```python
from build123d import *

# Parameters (mm, degrees)
F0_W     = 88.9
F0_H     = 25.4
F1_DEPTH = 3.175
F2_R     = 3.5
F3_DEPTH = 10.16
F4_R     = 1.9685
F5_DEPTH = 25.4
F6_W     = 4.374
F6_H     = 25.4
F7_DEPTH = 20.32


with BuildPart() as f1:
    # F0 (on Top) → F1 (new body)
    with BuildSketch(Plane.XY):
        Rectangle(F0_W, F0_H)
    extrude(amount=F1_DEPTH)

    # F2 (on face) → F3 (join)
    with BuildSketch(Plane.XY.offset(3.175)):
        with Locations((40.95, 0)):
            Circle(F2_R)
    extrude(amount=F3_DEPTH)

    # F4 (on face) → F5 (cut)
    with BuildSketch(Plane.XY.offset(3.175)):
        with Locations((3.612, 0)):
            Circle(F4_R)
    extrude(amount=-F5_DEPTH, mode=Mode.SUBTRACT)

    # F6 (on face) → F7 (join)
    with BuildSketch(Plane.XY.offset(3.175)):
        with Locations((-42.263, 0)):
            Rectangle(F6_W, F6_H)
    extrude(amount=F7_DEPTH)


solid = f1.part
```
Build history of the part. All positions in model axes, mm. A direction names the side the tool comes from. Round coordinates to 2 decimals unless told otherwise and drop trailing zeros. Order: outer loops, then holes, each group sorted by start corner. A loop starts at its lowest first (then second) coordinate and runs counter-clockwise, first axis right, second up. Notation, with made-up numbers: (11.5, 10) -> (16.5, 10) arc R33 ccw to (16.5, 46) -> close; hole circle Ø4 at (-24, 37). An arc over 180 degrees is marked (long way). Answer in a Markdown table with one row per item.
1) Band-saw the part on B-B on z = 7.25. Give the cut face in (x, y), and give its area (3 significant figures).
Values:
| item | result |
|---|---|
| outline | (-44.45, -12.7) -> (-40.08, -12.7) -> (-40.08, 12.7) -> (-44.45, 12.7) -> close; circle Ø7 at (40.95, 0) |
| area | 150 mm2 |
2) Band-saw the part on A-A on x = 2.5. Give the cut face in (y, z) (3 decimals), and give its area (3 significant figures).
Values:
| item | result |
|---|---|
| outline | (-12.7, 0) -> (-1.624, 0) -> (-1.624, 3.175) -> (-12.7, 3.175) -> close; (1.624, 0) -> (12.7, 0) -> (12.7, 3.175) -> (1.624, 3.175) -> close |
| area | 70.3 mm2 |
3) Band-saw the part on D-D on x = 40.95. Give the cut face in (y, z) (3 decimals), and give its area (3 significant figures).
Values:
| item | result |
|---|---|
| outline | (-12.7, 0) -> (12.7, 0) -> (12.7, 3.175) -> (3.5, 3.175) -> (3.5, 13.335) -> (-3.5, 13.335) -> (-3.5, 3.175) -> (-12.7, 3.175) -> close |
| area | 152 mm2 |
4) Which spindle directions (+Z, -Z, +X, -X, +Y, -Y) get a long thin tool onto all of the face, cutting with end or side? Do faces 1 (the flat face through (-40.076, 0, 13)), 2 (the flat face through (41, 0, 13.335)), 3 (the flat face through (-1, 0, 0)). Say none if no direction does.
Values:
| item | result |
|---|---|
| face 1 | +Z, +Y, -Y |
| face 2 | +Z, +X, +Y, -Y |
| face 3 | -Z, +X, -X, +Y, -Y |
5) Wall check: L1, parallel to Z at x = -16, y = 3 (3 decimals); L2, parallel to X at y = -7.5, z = 7.25; L3, parallel to X at y = 1, z = 9.5. Give the ranges that are in metal, low to high.
Values:
| item | result |
|---|---|
| L1 | 0 to 3.175 |
| L2 | -44.45 to -40.08 |
| L3 | -44.45 to -40.08, 37.6 to 44.3 |
6) Band-saw the part on C-C on y = -1. Give the cut face in (x, z) (3 decimals).
Values:
| item | result |
|---|---|
| outline | (-44.45, 0) -> (1.916, 0) -> (1.916, 3.175) -> (-40.076, 3.175) -> (-40.076, 23.495) -> (-44.45, 23.495) -> close; (5.308, 0) -> (44.45, 0) -> (44.45, 3.175) -> (44.304, 3.175) -> (44.304, 13.335) -> (37.596, 13.335) -> (37.596, 3.175) -> (5.308, 3.175) -> close |
7) Mould opens along Y. For faces 4 (the cylindrical face through (5.43, -0.75, 1.61)), 5 (the flat face through (2, -3, 3.175)), 6 (the cylindrical face through (44.29, 1.05, 8.18)) say: released by +Y, released by -Y, zero draft, split by the parting line, or undercut.
Values:
| item | result |
|---|---|
| face 4 | undercut |
| face 5 | zero draft |
| face 6 | split by the parting line |
8) Pin check, flat tips, straight feed: P1, Ø12.5, axis at x = -14, y = -2.5, coming from the +Z side (3 decimals); P2, Ø6, axis at y = 5.5, z = 9, coming from the +X side; P3, Ø7.5, axis at x = 39.5, y = 1.5, coming from the +Z side (3 decimals). Stop position of each tip, or through.
Values:
| item | result |
|---|---|
| P1 | z = 3.175 |
| P2 | x = 43.4 |
| P3 | z = 13.335 |
